Here's the drawing with two shaded views (mm, measured from the low corner). I have some questions. A direction names the side the tool comes from. Round coordinates to 2 decimals unless told otherwise and drop trailing zeros. Write each loop counter-clockwise with the first axis right and the second up, starting at its lowest first coordinate (ties: lowest second). Pieces come first, ordered by that corner, then holes. Notation, with made-up numbers: M -10,-31.75 L 25,-31.75 A23 ccw 25,-3.75 Z; hole C -24,21 d7. An arc over 180 degrees is marked long. Answer as a JSON object with one key per item and string values. Group by question number.
1) I'm going to push flat-ended pins straight in: pin 1 Ø3 at (x, y) = (165.5, 50) entering from -Z; pin 2 Ø10 at (x, y) = (101, 61) entering from -Z; pin 3 Ø5 at (x, y) = (69.5, 55.5) entering from -Z; pin 4 Ø10 at (x, y) = (30, 20) entering from -Z. Where does each tip first touch, or does it pass through?
2) Suppose I cut it at B-B, the plane x = 30. Write out the boundary of the cut face in (y, z).
3) Suppose I cut it at C-C, the plane z = 30. Write out the boundary of the cut face in (x, y), and give its area (3 significant figures).
4) Suppose I cut it at A-A, the plane y = 20. Write out the boundary of the cut face in (x, z).
5) If we mould it in two halves opening along X, with no side actions, what happens to the marked faces 3, 4 and 5? For each: +X half, -X half, draft (parallel to the pull), parting line (faces both ways), or undercut.
6) Please list where these lines run through material, in increasing order: L1, parallel to Y at x = 30, z = 45; L2, parallel to X at y = 20, z = 34; L3, parallel to Y at x = 35, z = 10. Write a range as [from, to].
7) On a 3-axis mill with a long thin cutter (end or side, diameter ignored), from which of +Z, -Z, +X, -X, +Y, -Y can I reach the whole of each face in a straight line? I mean the marked faces 1 and 2. Say none if no direction works.
8) Suppose I cut it at D-D, the plane y = 50. Write out the boundary of the cut face in (x, z), and give its area (3 significant figures).
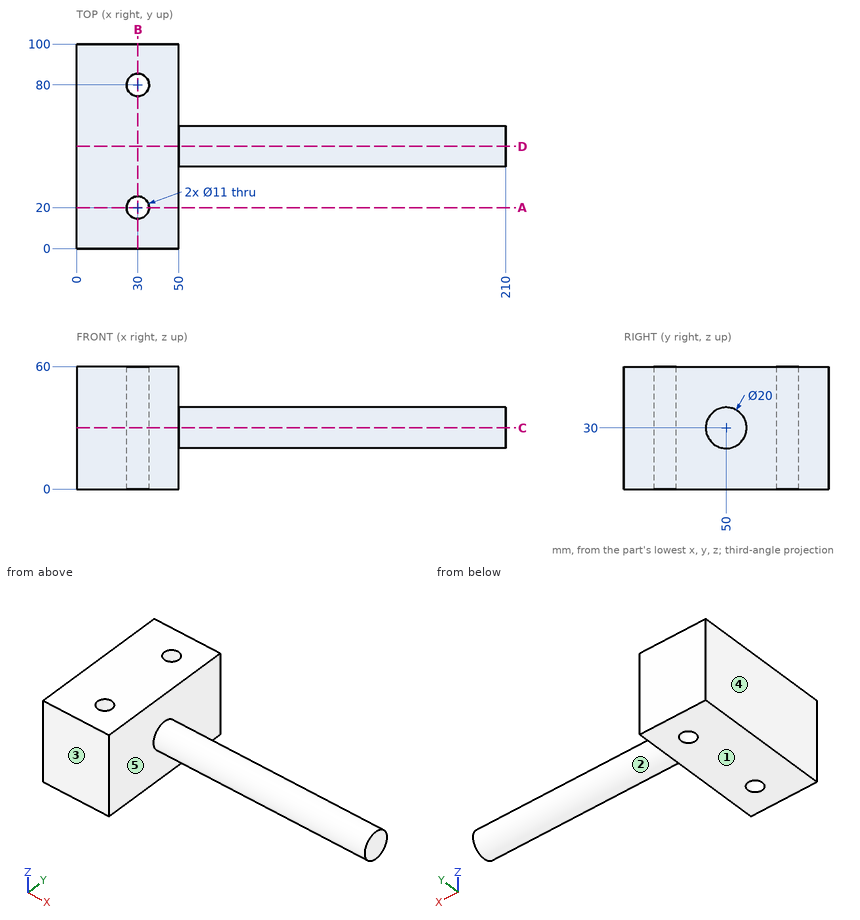
Results:
{
 "1": {"pin 1": "z = 20", "pin 2": "z = 22", "pin 3": "z = 20.46", "pin 4": "through"},
 "2": {"outline": "M 0,0 L 14.5,0 L 14.5,60 L 0,60 Z; M 25.5,0 L 74.5,0 L 74.5,60 L 25.5,60 Z; M 85.5,0 L 100,0 L 100,60 L 85.5,60 Z"},
 "3": {"outline": "M 0,0 L 50,0 L 50,40 L 210,40 L 210,60 L 50,60 L 50,100 L 0,100 Z; hole C 30,20 d11; hole C 30,80 d11", "area": "8,010 mm^2"},
 "4": {"outline": "M 0,0 L 24.5,0 L 24.5,60 L 0,60 Z; M 35.5,0 L 50,0 L 50,60 L 35.5,60 Z"},
 "5": {"face 3": "draft", "face 4": "-X half", "face 5": "+X half"},
 "6": {"L1": "[0, 14.5], [25.5, 74.5], [85.5, 100]", "L2": "[0, 24.5], [35.5, 50]", "L3": "[0, 17.71], [22.29, 77.71], [82.29, 100]"},
 "7": {"face 1": "-Z, +X, -X, +Y, -Y", "face 2": "+X"},
 "8": {"outline": "M 0,0 L 50,0 L 50,20 L 210,20 L 210,40 L 50,40 L 50,60 L 0,60 Z", "area": "6,200 mm^2"}
}
